from build123d import *

# Parameters (mm, degrees)
SKETCH1_R           = 1.42
SKETCH1_R_2         = 1.5
BOSS_EXTRUDE1_DEPTH = 3
CUT_EXTRUDE1_DEPTH  = 10
SKETCH3_R           = 1.25
CUT_EXTRUDE2_DEPTH  = 4
FILLET3_R           = 10
FILLET5_R           = 10
FILLET6_R           = 10


with BuildPart() as part:
    # Sketch1 → Boss-Extrude1 (new body)
    with BuildSketch(Plane(origin=(0, 0, 0), x_dir=(1, 0, 0), z_dir=(0, 1, 0))):
        with BuildLine():
            ThreePointArc((133.875699804, 40.34048493), (126.122977609, 46.855267092), (116.497088404, 50))
            Line((116.497088404, 50), (107.768405602, 58.234688612))
            Line((107.768405602, 58.234688612), (-44.546790917, 58.234688612))
            Line((-44.546790917, 58.234688612), (-53.27547372, 50))
            Line((-53.27547372, 50), (-60.834293515, 50))
            Line((-60.834293515, 50), (-79.287118585, 15.140440013))
            ThreePointArc((-79.287118585, 15.140440013), (-70.265146029, -8.871003651), (-47.526969146, 3))
            Line((-47.526969146, 3), (90.594512312, 3))
            ThreePointArc((90.594512312, 3), (97.400879011, -9.399948213), (110.470105416, -3.988787107))
            Line((110.470105416, -3.988787107), (136.480218576, -3.988787107))
            ThreePointArc((136.480218576, -3.988787107), (150.979390144, -8.686037245), (154.629343476, 6.111529301))
            Line((154.629343476, 6.111529301), (133.875699804, 40.34048493))
        make_face()
        with Locations(Location((145.916308107, 0.41174787, 0), (0, 0, 270))):
            Circle(SKETCH1_R, mode=Mode.SUBTRACT)
        with Locations(Location((100.916308107, 0, 0), (0, 0, 270))):
            Circle(SKETCH1_R, mode=Mode.SUBTRACT)
        with Locations(Location((-64.083691893, 0, 0), (0, 0, 270))):
            Circle(SKETCH1_R_2, mode=Mode.SUBTRACT)
    extrude(amount=BOSS_EXTRUDE1_DEPTH)

    # Sketch2 → Cut-Extrude1 (cut)
    with BuildSketch(Plane(origin=(0, 3, 0), x_dir=(1, 0, 0), z_dir=(0, 1, 0))):
        with BuildLine():
            Line((67.972610999, 16.705365669), (-21.876516484, 16.705365669))
            ThreePointArc((-21.876516484, 16.705365669), (-29.906807538, 24.735656723), (-21.876516484, 32.765947778))
            Line((-21.876516484, 32.765947778), (67.972610999, 32.765947778))
            ThreePointArc((67.972610999, 32.765947778), (76.002902053, 24.735656723), (67.972610999, 16.705365669))
        make_face()
    extrude(amount=-CUT_EXTRUDE1_DEPTH, mode=Mode.SUBTRACT)

    # Sketch3 → Cut-Extrude2 (cut)
    with BuildSketch(Plane(origin=(0, 3, 0), x_dir=(1, 0, 0), z_dir=(0, 1, 0))):
        with Locations(Location((-4.515015694, 7, 0), (0, 0, 270))):
            Circle(SKETCH3_R)
        with Locations(Location((68.446888698, 7, 0), (0, 0, 270))):
            Circle(SKETCH3_R)
        with Locations(Location((-4.515015694, 53.518369915, 0), (0, 0, 270))):
            Circle(SKETCH3_R)
        with Locations(Location((69.48070481, 53.518369915, 0), (0, 0, 270))):
            Circle(SKETCH3_R)
    extrude(amount=-CUT_EXTRUDE2_DEPTH, mode=Mode.SUBTRACT)

    # Fillet3
    fillet3_edges = [part.edges().sort_by_distance(p)[0] for p in [
        (110.470105416, 1.5, 3.988787107),
        (90.594512312, 1.5, -3),
        (-47.526969146, 1.5, -3),
        (136.480218576, 1.5, 3.988787107),
    ]]
    fillet(fillet3_edges, radius=FILLET3_R)

    # Fillet5
    fillet5_edges = [part.edges().sort_by_distance(p)[0] for p in [
        (-53.27547372, 1.5, -50),
        (-44.546790917, 1.5, -58.234688612),
        (107.768405602, 1.5, -58.234688612),
        (116.497088404, 1.5, -50),
    ]]
    fillet(fillet5_edges, radius=FILLET5_R)

    # Fillet6
    fillet6_edges = [part.edges().sort_by_distance(p)[0] for p in [
        (-60.834293515, 1.5, -50),
    ]]
    fillet(fillet6_edges, radius=FILLET6_R)


solid = part.part
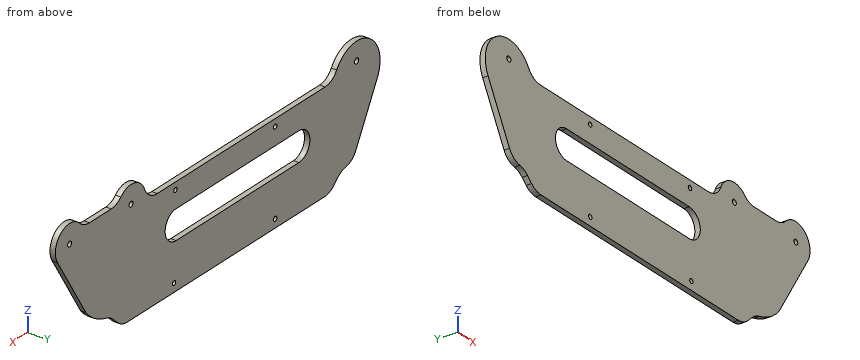
Verification items for the finished model (mm, model axes). Coordinates: 2 decimals unless noted, no trailing zeros. Order: outer loops, then holes, each group sorted by start corner. A loop starts at its lowest first (then second) coordinate and runs counter-clockwise, first axis right, second up.
1. Sectioned sample at B-B, the plane y = 0.75. Give the number of separate pieces and of enclosed holes in the cut face, and give its area (3 significant figures).
Results found:
separate pieces: 1
enclosed holes: 8
area: 10,700 mm2
2. Sectioned sample at C-C, the plane x = 128. Record the cut outline in (y, z), and give its area (3 significant figures).
Results found:
outline: (0, -45.71) - (3, -45.71) - (3, 3.99) - (0, 3.99) - close
area: 149 mm2
3. Sectioned sample at A-A, the plane x = 56. Record the cut outline in (y, z).
Results found:
outline: (0, -58.23) - (3, -58.23) - (3, -32.77) - (0, -32.77) - close; (0, -16.71) - (3, -16.71) - (3, -3) - (0, -3) - close
4. Go/stop test with flat-tipped pins: pin 1 Ø1.5 at (x, y) = (123, 1) entering from +Z; pin 2 Ø1.5 at (x, z) = (-4.52, -7) entering from +Y; pin 3 Ø1 at (y, z) = (2, -29) entering from -X. Record where each tip stops, or that it passes through.
Results found:
pin 1: stops at z = 3.99
pin 2: passes through
pin 3: stops at x = -72.22
5. Scan lines: line 1 (Z direction, x = 43.5, y = 1.85); line 2 (X direction, y = 1.15, z = 5.5); line 3 (X direction, y = 0.6, z = -22.5). Record each from-to range of solid material in increasing order.
Results found:
line 1: z = -58.23 to -32.77, -16.71 to -3
line 2: x = -75.72 to -52.58, 92.25 to 110.17, 136.74 to 154.49
line 3: x = -75.39 to -29.59, 75.69 to 144.69
